Model file for the job. Use its own axes, mm. A direction names the side the tool comes from. Coordinates: 2 decimals unless noted, no trailing zeros. Order: outer loops, then holes, each group sorted by start corner. A loop starts at its lowest first (then second) coordinate and runs counter-clockwise, first axis right, second up.
from build123d import *

# Parameters (mm, degrees)
F2_W            = 7.5
F2_H            = 8
F3_DEPTH        = 3
F3_COPIES_COUNT = 4
F4_R            = 5


# Not quite as in the source:
# - a pattern or mirror of a feature is missing from the dataset's text; its kind, count and spacing are read off the source's solid


with BuildPart() as f1:
    # F0 (on Front) → F1 (revolve)
    with BuildSketch(Plane.XZ):
        Polygon((23.9476348052, 3), (24, 0), (30, 0), (30, 3), align=None)
        Polygon((20.9525509577, 59.9908617094), (21.9473301491, 3), (23.9476348052, 3), (22.9528556138, 59.9908617094), align=None)
        Polygon((21.9473301491, 3), (21.9996953439, 0), (24, 0), (23.9476348052, 3), align=None)
    revolve(axis=Axis((0, 0, 53.7638920359), (0, 0, -1)))

    # F2 (on face) → F3 (join)
    with BuildSketch(Plane(origin=(0, 0, 0), x_dir=(1, 0, 0), z_dir=(0, 0, -1))):
        with Locations((0, 30)):
            Rectangle(F2_W, F2_H)
    f3 = extrude(amount=-F3_DEPTH)

    # F3_copies: F3 ×4 about axis
    f3_copies_axis = Axis((0, 0, 0), (0, 0, 1))
    for i in range(1, F3_COPIES_COUNT):
        add(f3.rotate(f3_copies_axis, i * 360 / F3_COPIES_COUNT))

    # F4
    f4_edges = [f1.edges().sort_by_distance(p)[0] for p in [
        (-23.947635, 0, 3),
        (-21.999695, 0, 0),
    ]]
    fillet(f4_edges, radius=F4_R)


solid = f1.part
Q1. Probe line 1 (X direction, y = 3, z = 39); line 2 (Z direction, x = -7.5, y = 29); line 3 (Y direction, x = 19, z = 23.5). List the from-to ranges inside material, lowest first.
Established:
line 1: x = -23.13 to -21.11, 21.11 to 23.13
line 2: z = 0 to 3
line 3: y = -13.98 to -10.25, 10.25 to 13.98
Q2. Cut at A-A, the plane z = 13. List the corners of the cut face in (x, y).
Established:
outline: circle Ø47.55 at (0, 0); hole circle Ø43.55 at (0, 0)
Q3. Mould opens along X. For faces 6 (the face through (-32, -3.75, 1)), 7 (the face through (21.016, 21.408, 1.521)), 8 (the face through (-4.65, 20.93, 32.07)) say: pulls with the +X half, pulls with the -X half, needs draft (parallel to the pull), parting line crosses it, or undercut.
Established:
face 6: needs draft
face 7: pulls with the +X half
face 8: undercut
Q4. Drop flat-ended pins along their axis: P1, Ø10, axis at y = -20.5, z = 9, coming from the +X side; P2, Ø2, axis at x = 2.5, z = 28.5, coming from the -Y side; P3, Ø1.5, axis at x = -31.5, z = 2, coming from the -Y side. Give the stop position or say it passes through.
Established:
P1: stops at x = 18.12
P2: stops at y = -23.46
P3: stops at y = -3.75
Q5. Which spindle directions (+Z, -Z, +X, -X, +Y, -Y) get a long thin tool onto all of the face, cutting with end or side? Do faces 1 (the face through (3.75, 32, 1)), 2 (the face through (-3.75, -32, 1)), 3 (the face through (-18, -23, 3)), 4 (the face through (3.75, -32, 1)), 5 (the face through (-3.75, 32, 1)). Say none if no direction does.
Established:
face 1: +Z, -Z, +X, +Y
face 2: +Z, -Z, -X, -Y
face 3: +Z
face 4: +Z, -Z, +X, -Y
face 5: +Z, -Z, -X, +Y
Q6. Cut at B-B, the plane z = 22.5. List the corners of the cut face in (x, y), plus the area to 3 significant figures.
Established:
outline: circle Ø47.21 at (0, 0); hole circle Ø43.21 at (0, 0)
area: 284 mm2
